from build123d import *

# Parameters (mm, degrees)
F0_W      = 143
F0_H      = 72.17
F1_DEPTH  = 7.17
F2_W      = 72.17
F2_H      = 19.87
F3_DEPTH  = 6.35
F4_W      = 72.17
F4_H      = 19.87
F5_DEPTH  = 6.35
F6_W      = 143
F6_H      = 6.3621380544
F7_DEPTH  = 6.35
F8_W      = 143
F8_H      = 6.358533836
F9_DEPTH  = 6.35
F10_W     = 155.7
F10_H     = 19.87
F11_DEPTH = 6.35
F12_W     = 143
F12_H     = 7.17
F13_DEPTH = 65.811466164
F14_W     = 143
F14_H     = 7.17
F15_DEPTH = 6.35
F16_W     = 65.811466164
F16_H     = 6.35
F17_DEPTH = 3.81
F18_W     = 65.8105651094
F18_H     = 6.35
F19_DEPTH = 3.81
F20_W     = 65.811466164
F20_H     = 6.35
F21_DEPTH = 3.81
F22_W     = 65.8105651094
F22_H     = 6.35
F23_DEPTH = 3.81
F24_W     = 52.8727266937
F24_H     = 7.17
F25_DEPTH = 25.4
F26_R     = 1.27
F27_DEPTH = 149.35


with BuildPart() as f1:
    # F0 (on Top) → F1 (new body)
    with BuildSketch(Plane.XY):
        Rectangle(F0_W, F0_H)
    extrude(amount=F1_DEPTH)

    # F2 (on face) → F3 (join)
    with BuildSketch(Plane.YZ.offset(71.5)):
        with Locations((0, 3.585)):
            Rectangle(F2_W, F2_H)
    extrude(amount=F3_DEPTH)

    # F4 (on face) → F5 (join)
    with BuildSketch(Plane(origin=(-71.5, 0, 0), x_dir=(0, -1, 0), z_dir=(-1, 0, 0))):
        with Locations((0, 3.585)):
            Rectangle(F4_W, F4_H)
    extrude(amount=F5_DEPTH)

    # F6 (on face) → F7 (join)
    with BuildSketch(Plane.XY.offset(7.17)):
        with Locations((0, 32.9039309728)):
            Rectangle(F6_W, F6_H)
    extrude(amount=F7_DEPTH)

    # F8 (on face) → F9 (join)
    with BuildSketch(Plane(origin=(0, 0, 0), x_dir=(1, 0, 0), z_dir=(0, 0, -1))):
        with Locations((0, -32.905733082)):
            Rectangle(F8_W, F8_H)
    extrude(amount=F9_DEPTH)

    # F10 (on face) → F11 (join)
    with BuildSketch(Plane(origin=(0, 36.085, 0), x_dir=(-1, 0, 0), z_dir=(0, 1, 0))):
        with Locations((0, 3.585)):
            Rectangle(F10_W, F10_H)
    extrude(amount=F11_DEPTH)

    # F12 (on face) → F13 (cut, through all)
    with BuildSketch(Plane.XZ.offset(36.085)):
        with Locations((0, 3.585)):
            Rectangle(F12_W, F12_H)
    extrude(amount=-F13_DEPTH, mode=Mode.SUBTRACT)

    # F14 (on face) → F15 (cut)
    with BuildSketch(Plane.XZ.offset(-29.726466164)):
        with Locations((0, 3.585)):
            Rectangle(F14_W, F14_H)
    extrude(amount=-F15_DEPTH, mode=Mode.SUBTRACT)

    # F16 (on face) → F17 (join)
    with BuildSketch(Plane(origin=(71.5, 0, 0), x_dir=(0, -1, 0), z_dir=(-1, 0, 0))):
        with Locations((3.179266918, -3.175)):
            Rectangle(F16_W, F16_H)
    extrude(amount=F17_DEPTH)

    # F18 (on face) → F19 (join)
    with BuildSketch(Plane(origin=(71.5, 0, 0), x_dir=(0, -1, 0), z_dir=(-1, 0, 0))):
        with Locations((3.1797174453, 10.345)):
            Rectangle(F18_W, F18_H)
    extrude(amount=F19_DEPTH)

    # F20 (on face) → F21 (join)
    with BuildSketch(Plane.YZ.offset(-71.5)):
        with Locations((-3.179266918, -3.175)):
            Rectangle(F20_W, F20_H)
    extrude(amount=F21_DEPTH)

    # F22 (on face) → F23 (join)
    with BuildSketch(Plane.YZ.offset(-71.5)):
        with Locations((-3.1797174453, 10.345)):
            Rectangle(F22_W, F22_H)
    extrude(amount=F23_DEPTH)

    # F24 (on face) → F25 (cut)
    with BuildSketch(Plane.YZ.offset(77.85)):
        with Locations((3.4307548776, 3.585)):
            Rectangle(F24_W, F24_H)
    extrude(amount=-F25_DEPTH, mode=Mode.SUBTRACT)

    # F26 (on face) → F27 (cut, through all)
    with BuildSketch(Plane(origin=(-77.85, 0, 0), x_dir=(0, -1, 0), z_dir=(-1, 0, 0))):
        with Locations((-7.3689044776, 5.0491553406)):
            Circle(F26_R)
        with Locations((8.3790955224, 5.0491553406)):
            Circle(F26_R)
    extrude(amount=-F27_DEPTH, mode=Mode.SUBTRACT)


solid = f1.part
Input: part model. Units: mm. Frame: model coordinates. A direction names the side the tool comes from. Give positions to 0.01 mm unless a question says otherwise; leave off trailing zeros. Write each loop counter-clockwise with the first axis right and the second up, starting at its lowest first coordinate (ties: lowest second). Pieces come first, ordered by that corner, then holes. Notation, with made-up numbers: M 18,15 L 29,15 A31 ccw 29,47 Z; hole C 30,-39.5 d7. An arc over 180 degrees is marked long. Write item = value, one per line. Start each with the question number.
1) Draft query along Y for faces 1 (the flat face through (14, 32, 7.17)), 2 (the flat face through (-1, 29.726, -3)), 3 (the flat face through (71.5, 33, 4)). Return one class per face: +Y half, -Y half, draft (parallel to the pull), parting line (faces both ways), or undercut.
2) Material intervals for line 1 along X through (y, z) = (-20, -5.25); line 2 along Z through (x, y) = (-67, 35.5); line 3 along Y through (x, z) = (-5, 7.5) (3 decimals), sorted ascending. Write a range as [from, to].
3) Cut plane C-C on x = 26.5. Return the cut outline in (y, z) (3 decimals), then the cut area to 3 significant figures.
4) Reachability of faces 4 (the flat face through (75, 29.867, 4)), 5 (the flat face through (14, 32, 0)), 6 (the flat face through (71.5, -30, 4)) from +Z, -Z, +X, -X, +Y, -Y: full face, straight path, thin tool, end or side. Return the list, or none.
5) Cut plane B-B on z = -2. Return the cut outline in (x, y) (3 decimals), then the cut area to 3 significant figures.
6) Cut plane A-A on y = -2.5. Return the cut outline in (x, z).
7) First-contact query: pin 1 Ø10 at (x, z) = (17.5, 9) entering from -Y; pin 2 Ø1.5 at (x, z) = (-24.5, 3) entering from -Y; pin 3 Ø3 at (y, z) = (-8.38, 5.05) entering from +X; pin 4 Ø8 at (x, y) = (-59, 25.5) entering from +Z. Flat tips, straight axial feed; report the tip coordinate or a pass-through.
Solved:
q1.face_1 = undercut
q1.face_2 = -Y half
q1.face_3 = draft
q2.line_1 = [-77.85, -67.69], [67.69, 77.85]
q2.line_2 = [-6.35, 0], [7.17, 13.52]
q2.line_3 = [29.723, 42.435]
q3.outline = M 29.723,7.17 L 36.076,7.17 L 36.076,0 L 29.726,0 L 29.726,-6.35 L 42.435,-6.35 L 42.435,13.52 L 29.723,13.52 Z
q3.area = 207 mm2
q4.face_4 = +X
q4.face_5 = none
q4.face_6 = -Y
q5.outline = M -77.85,-36.085 L -67.69,-36.085 L -67.69,29.726 L 67.69,29.726 L 67.69,-36.085 L 77.85,-36.085 L 77.85,42.435 L -77.85,42.435 Z
q5.area = 3,320 mm2
q6.outline = M -77.85,-6.35 L -67.69,-6.35 L -67.69,0 L -71.5,0 L -71.5,7.17 L -67.69,7.17 L -67.69,13.52 L -77.85,13.52 Z; M 67.69,-6.35 L 77.85,-6.35 L 77.85,0 L 67.69,0 Z; M 67.69,7.17 L 77.85,7.17 L 77.85,13.52 L 67.69,13.52 Z
q7.pin_1 = 29.72
q7.pin_2 = 36.08
q7.pin_3 = -71.5
q7.pin_4 = through
